```python
from build123d import *

# Parameters (mm, degrees)
F3_DEPTH      = 27.501
F3_DEPTH_BACK = 27.501
F4_R          = 7.5
F5_DEPTH      = 24.2238989074
F7_R          = 6
F8_DEPTH      = 2
F8_DEPTH_BACK = 12.2238989074
F9_SIZE       = 0.5


with BuildPart() as f1:
    # F0 (on Front) → F1 (revolve)
    with BuildSketch(Plane.XZ):
        with BuildLine():
            Line((27.5, 0), (0, 0))
            Line((0, 0), (0, -43.3184476327))
            ThreePointArc((0, -43.3184476327), (12.0343671506, -39.2926145056), (19.2238989074, -28.8358483611))
            Line((19.2238989074, -28.8358483611), (27.5, 0))
        make_face()
    revolve(axis=Axis((0, 0, 4.3592059342), (0, 0, 1)))

    # F2 (on Front) → F3 (cut, two sides)
    with BuildSketch(Plane.XZ) as f3_sk:
        Polygon((0, -43.3184476327), (12, -43.3184476327), (12, -3.3184476327), (0, -3.3184476327), (-12, -3.3184476327), (-12, -43.3184476327), align=None)
    extrude(amount=-F3_DEPTH, mode=Mode.SUBTRACT)
    extrude(f3_sk.sketch, amount=F3_DEPTH_BACK, mode=Mode.SUBTRACT)

    # F4 (on Right) → F5 (join, through all)
    with BuildSketch(Plane.YZ):
        with Locations((0, -23.3184476327)):
            Circle(F4_R)
    extrude(amount=F5_DEPTH)

    # F6: F1 across plane


with BuildPart() as f1_1:
    add(f1.part)
    add(f1.part.mirror(Plane.YZ))

    # F7 (on face) → F8 (join, two sides)
    with BuildSketch(Plane.YZ.offset(24.2238989074)) as f8_sk:
        with Locations((0, -23.3184476327)):
            Circle(F7_R)
    extrude(amount=F8_DEPTH)
    extrude(f8_sk.sketch, amount=-F8_DEPTH_BACK)

    # F9
    f9_edges = [f1_1.edges().sort_by_distance(p)[0] for p in [
        (26.223899, -6, -23.318448),
        (-24.223899, -7.5, -23.318448),
        (24.223899, -7.5, -23.318448),
    ]]
    chamfer(f9_edges, length=F9_SIZE)


solid = f1_1.part
```
Read the model definition and answer for the solid it produces. Units are mm, in the model's axes. A direction names the side the tool comes from. Give positions to 0.01 mm unless a question says otherwise; leave off trailing zeros. Loops run counter-clockwise (first coordinate to the right, second up) from the corner with the lowest first, then second, coordinate; pieces in that order, holes last.
Item 1: The mould has two halves that part along Z. Classify faces 5 (the flat face through (26.224, 0, -23)), 6 (the cylindrical face through (21.67, -1.63, -30.64)), 7 (the flat face through (0, 0, 0)): released by +Z, released by -Z, zero draft, split by the parting line, or undercut.
Item 2: For faces 1 (the flat face through (-12, 0, -13)), 2 (the flat face through (24.224, 6, -21)), 3 (the flat face through (-24.224, 0, -23)), 4 (the flat face through (0, 0, -3.318)), determine the directions among +Z, -Z, +X, -X, +Y, -Y from which every point of the face is accessible in a straight line to the end or side of a thin tool.
Item 3: Find the intervals of material crossed by line 1 along X through (y, z) = (1, -13); line 2 along X through (y, z) = (-3.5, -26.5); line 3 along X through (y, z) = (19, -6.5), in increasing order.
Item 4: The part is cut by section B-B (z = -8). Write down the section's boundary in (x, y).
Item 5: The part is cut by section A-A (y = 0). Write down the section's boundary in (x, z).
Item 6: Each of these flat-tipped pins is pushed along its axis until it touches: pin 1 Ø4 at (x, z) = (16.5, -11.5) entering from +Y; pin 2 Ø12 at (x, y) = (9, 12.5) entering from -Z; pin 3 Ø15.5 at (y, z) = (0.5, -21.5) entering from +X. Where does it stop, or does it pass through?
Taken from the geometry:
1. face 5: zero draft
1. face 6: undercut
1. face 7: released by +Z
2. face 1: none
2. face 2: +X
2. face 3: -Z, -X, +Y, -Y
2. face 4: +Y, -Y
3. line 1: x = -23.75 to -12, 12 to 23.75
3. line 2: x = -24.22 to 26.22
3. line 3: x = -17.21 to -12, 12 to 17.21
4. outline: (-12, -22.16) - (-12, 22.16) arc R25.2 ccw to start; (12, -22.16) arc R25.2 ccw to (12, 22.16) - close
5. outline: (-27.5, 0) - (-22.96, -15.82) - (-23.72, -15.82) - (-24.22, -16.32) - (-24.22, -30.32) - (-23.72, -30.82) - (-18.54, -30.82) arc R20 ccw to (-12, -39.32) - (-12, -30.82) - (12, -30.82) - (12, -39.32) arc R20 ccw to (18.54, -30.82) - (23.72, -30.82) - (24.22, -30.32) - (24.22, -29.32) - (25.72, -29.32) - (26.22, -28.82) - (26.22, -17.82) - (25.72, -17.32) - (24.22, -17.32) - (24.22, -16.32) - (23.72, -15.82) - (22.96, -15.82) - (27.5, 0) - close; hole (-12, -15.82) - (12, -15.82) - (12, -3.32) - (-12, -3.32) - close
6. pin 1: stops at y = 19.54
6. pin 2: stops at z = -37.55
6. pin 3: stops at x = 26.22
